from build123d import *

# Parameters (mm, degrees)
BOX021_W          = 7
BOX021_H          = 3
BOX021_DEPTH      = 7
CHAMFER010_SIZE   = 1
BOX020_W          = 7
BOX020_H          = 3
BOX020_DEPTH      = 7
CHAMFER011_SIZE   = 1
CYLINDER026_R     = 2.5
CYLINDER026_DEPTH = 5
CYLINDER027_R     = 2.5
CYLINDER027_DEPTH = 5
CYLINDER029_R     = 0.85
CYLINDER029_DEPTH = 18
CYLINDER028_R     = 0.85
CYLINDER028_DEPTH = 18
BOX022_W          = 10
BOX022_H          = 20
BOX022_DEPTH      = 3
CHAMFER012_SIZE   = 1
CHAMFER013_SIZE   = 1


with BuildPart() as chamfer010:
    # Box021 → Box021 (new body)
    with BuildSketch(Plane(origin=(-8, 7, 5), x_dir=(1, 0, 0), z_dir=(0, 0, 1))):
        with Locations((3.5, 1.5)):
            Rectangle(BOX021_W, BOX021_H)
    extrude(amount=BOX021_DEPTH)

    # Chamfer010
    chamfer010_edges = [chamfer010.edges().sort_by_distance(p)[0] for p in [
        (-8, 10, 8.5),
    ]]
    chamfer(chamfer010_edges, length=CHAMFER010_SIZE)


with BuildPart() as chamfer011:
    # Box020 → Box020 (new body)
    with BuildSketch(Plane(origin=(-8, -10, 5), x_dir=(1, 0, 0), z_dir=(0, 0, 1))):
        with Locations((3.5, 1.5)):
            Rectangle(BOX020_W, BOX020_H)
    extrude(amount=BOX020_DEPTH)

    # Chamfer011
    chamfer011_edges = [chamfer011.edges().sort_by_distance(p)[0] for p in [
        (-8, -10, 8.5),
    ]]
    chamfer(chamfer011_edges, length=CHAMFER011_SIZE)


with BuildPart() as cylinder026:
    # Cylinder026 → Cylinder026 (new body)
    with BuildSketch(Plane(origin=(-2.75, 3.25, 0), x_dir=(1, 0, 0), z_dir=(0, 0, 1))):
        Circle(CYLINDER026_R)
    extrude(amount=CYLINDER026_DEPTH)


with BuildPart() as fusion001001001011002006:
    # Cylinder027 → Cylinder027 (new body)
    with BuildSketch(Plane(origin=(-2.75, -3.25, 0), x_dir=(1, 0, 0), z_dir=(0, 0, 1))):
        Circle(CYLINDER027_R)
    extrude(amount=CYLINDER027_DEPTH)

    # Fusion001001001011002006: union Cylinder026
    add(cylinder026.part)


with BuildPart() as fusion001001001011002006_1:
    # Fusion001001001011002006 placement: moved
    add(fusion001001001011002006.part.moved(Location((0, 0, 12))))


with BuildPart() as cylinder029:
    # Cylinder029 → Cylinder029 (new body)
    with BuildSketch(Plane(origin=(-2.75, 3.25, 0), x_dir=(1, 0, 0), z_dir=(0, 0, 1))):
        Circle(CYLINDER029_R)
    extrude(amount=CYLINDER029_DEPTH)


with BuildPart() as fusion001001001011002005:
    # Cylinder028 → Cylinder028 (new body)
    with BuildSketch(Plane(origin=(-2.75, -3.25, 0), x_dir=(1, 0, 0), z_dir=(0, 0, 1))):
        Circle(CYLINDER028_R)
    extrude(amount=CYLINDER028_DEPTH)

    # Fusion001001001011002005: union Cylinder029
    add(cylinder029.part)


with BuildPart() as fusion001001001011002004002:
    # Box022 → Box022 (new body)
    with BuildSketch(Plane(origin=(-8, -10, 10.5), x_dir=(1, 0, 0), z_dir=(0, 0, 1))):
        with Locations((5, 10)):
            Rectangle(BOX022_W, BOX022_H)
    extrude(amount=BOX022_DEPTH)

    # Chamfer012
    chamfer012_edges = [fusion001001001011002004002.edges().sort_by_distance(p)[0] for p in [
        (-8, -10, 12),
        (-8, 10, 12),
    ]]
    chamfer(chamfer012_edges, length=CHAMFER012_SIZE)

    # Chamfer013
    chamfer013_edges = [fusion001001001011002004002.edges().sort_by_distance(p)[0] for p in [
        (-8, 0, 13.5),
        (-7.5, -9.5, 13.5),
        (-7.5, 9.5, 13.5),
        (-2.5, -10, 13.5),
        (-2.5, 10, 13.5),
    ]]
    chamfer(chamfer013_edges, length=CHAMFER013_SIZE)

    # Cut002008023012009006003002006002006002004004003: cut Fusion001001001011002005
    add(fusion001001001011002005.part, mode=Mode.SUBTRACT)


with BuildPart() as fusion001001001011002004002_1:
    # Cut002008023012009006003002006002006002004004003 placement: moved
    add(fusion001001001011002004002.part.moved(Location((0, 0, 0.5))))

    # Cut002008023012009006003002006002006002004004004: cut Fusion001001001011002006
    add(fusion001001001011002006_1.part, mode=Mode.SUBTRACT)


with BuildPart() as fusion001001001011002004002_2:
    # Cut002008023012009006003002006002006002004004004 placement: moved
    add(fusion001001001011002004002_1.part.moved(Location((0, 0, -0.25))))

    # Fusion001001001011002004002: union Chamfer010, Chamfer011
    add(chamfer010.part)
    add(chamfer011.part)


solid = fusion001001001011002004002_2.part
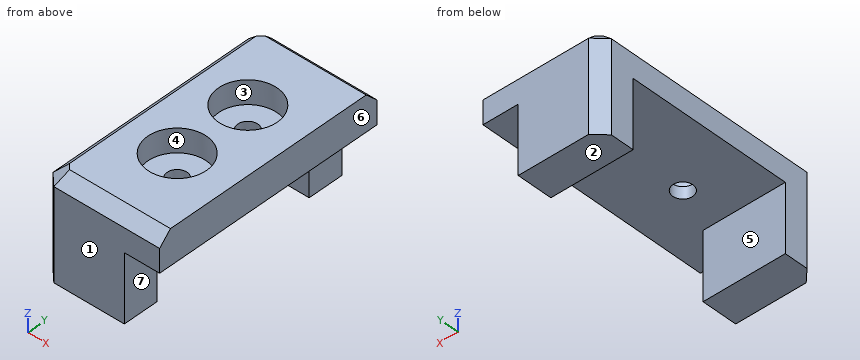
Input: part model. Units: mm. Frame: model coordinates. Face numbers are marked on the shaded views. A direction names the side the tool comes from. Give positions to 0.01 mm unless a question says otherwise; leave off trailing zeros. Order: outer loops, then holes, each group sorted by start corner. A loop starts at its lowest first (then second) coordinate and runs counter-clockwise, first axis right, second up. Notation, with made-up numbers: M 23.5,-31.75 L 53.5,-31.75 A20 cw 53.5,-16.75 Z; hole C 12,-35.5 d2. An arc over 180 degrees is marked long. Answer as a JSON object with one key per item and string values.
1. Cut plane D-D, the plane z = 12.5. Output: boundary loops of the cut face in (x, y), and give its area (3 significant figures).
Result sheet:
{"outline": "M -8,-9 L -7,-10 L 2,-10 L 2,10 L -7,10 L -8,9 Z; hole C -2.75,-3.25 d5; hole C -2.75,3.25 d5", "area": "160 mm²"}
2. Pull-direction query (Y, two-part tool) for the marked faces 1, 2 and 3; classes: +Y half, -Y half, draft (parallel to the pull), parting line (faces both ways), or undercut.
Result sheet:
{"face 1": "-Y half", "face 2": "draft", "face 3": "undercut"}
3. Cut plane C-C, the plane z = 9.75. Output: boundary loops of the cut face in (x, y).
Result sheet:
{"outline": "M -8,-9 L -7,-10 L -1,-10 L -1,-7 L -8,-7 Z; M -8,7 L -1,7 L -1,10 L -7,10 L -8,9 Z"}
4. First-contact query: P1, Ø4.5, axis at x = -2.75, y = 3.25, coming from the -Z side; P2, Ø1, axis at x = -2.75, y = -3.25, coming from the +Z side; P3, Ø2.5, axis at y = -9, z = 6.5, coming from the +X side. Flat tips, straight axial feed; report the tip coordinate or a pass-through.
Result sheet:
{"P1": "z = 10.75", "P2": "through", "P3": "x = -1"}
5. Cut plane A-A, the plane y = 3.25. Output: boundary loops of the cut face in (x, z), and give its area (3 significant figures).
Result sheet:
{"outline": "M -8,10.75 L -3.6,10.75 L -3.6,11.75 L -5.25,11.75 L -5.25,13.75 L -7,13.75 L -8,12.75 Z; M -1.9,10.75 L 2,10.75 L 2,13.75 L -0.25,13.75 L -0.25,11.75 L -1.9,11.75 Z", "area": "17.8 mm²"}
6. Cut plane B-B, the plane x = -2.75. Output: boundary loops of the cut face in (y, z), and give its area (3 significant figures).
Result sheet:
{"outline": "M -10,5 L -7,5 L -7,10.75 L -4.1,10.75 L -4.1,11.75 L -5.75,11.75 L -5.75,13.75 L -9,13.75 L -10,12.75 Z; M -2.4,10.75 L 2.4,10.75 L 2.4,11.75 L 0.75,11.75 L 0.75,13.75 L -0.75,13.75 L -0.75,11.75 L -2.4,11.75 Z; M 4.1,10.75 L 7,10.75 L 7,5 L 10,5 L 10,12.75 L 9,13.75 L 5.75,13.75 L 5.75,11.75 L 4.1,11.75 Z", "area": "70.1 mm²"}
7. Ray query, line 1 (Y direction, x = -2.75, z = 11.05); line 2 (Y direction, x = -2.75, z = 12.45); line 3 (Y direction, x = -4, z = 6.25). Return the intervals inside material, ascending. Write a range as [from, to].
Result sheet:
{"line 1": "[-10, -4.1], [-2.4, 2.4], [4.1, 10]", "line 2": "[-10, -5.75], [-0.75, 0.75], [5.75, 10]", "line 3": "[-10, -7], [7, 10]"}
8. Reachability of the marked faces 4, 5, 6 and 7 from +Z, -Z, +X, -X, +Y, -Y: full face, straight path, thin tool, end or side. Return the list, or none.
Result sheet:
{"face 4": "+Z", "face 5": "-Z, +X, -X", "face 6": "+Z, -Z, +X, +Y, -Y", "face 7": "-Z, +X, +Y, -Y"}
